```python
from build123d import *

# Parameters (mm, degrees)
SKETCH1_R           = 2.5
BOSS_EXTRUDE1_DEPTH = 1120


with BuildPart() as part:
    # Sketch1 → Boss-Extrude1 (new body)
    with BuildSketch(Plane.XY):
        with BuildLine():
            Line((2.839339828, 3.9), (-2.839339828, 3.9))
            Line((-2.839339828, 3.9), (-5.5, 6.560660172))
            Line((-5.5, 6.560660172), (-5.5, 8.2))
            Line((-5.5, 8.2), (-3.1, 8.2))
            Line((-3.1, 8.2), (-3.1, 9))
            Line((-3.1, 9), (-4.1, 10))
            Line((-4.1, 10), (-8.5, 10))
            ThreePointArc((-8.5, 10), (-9.560660172, 9.560660172), (-10, 8.5))
            Line((-10, 8.5), (-10, 4.1))
            Line((-10, 4.1), (-9, 3.1))
            Line((-9, 3.1), (-8.2, 3.1))
            Line((-8.2, 3.1), (-8.2, 5.5))
            Line((-8.2, 5.5), (-6.560660172, 5.5))
            Line((-6.560660172, 5.5), (-3.9, 2.839339828))
            Line((-3.9, 2.839339828), (-3.9, -2.839339828))
            Line((-3.9, -2.839339828), (-6.560660172, -5.5))
            Line((-6.560660172, -5.5), (-8.2, -5.5))
            Line((-8.2, -5.5), (-8.2, -3.1))
            Line((-8.2, -3.1), (-9, -3.1))
            Line((-9, -3.1), (-10, -4.1))
            Line((-10, -4.1), (-10, -8.5))
            ThreePointArc((-10, -8.5), (-9.560660172, -9.560660172), (-8.5, -10))
            Line((-8.5, -10), (-4.1, -10))
            Line((-4.1, -10), (-3.1, -9))
            Line((-3.1, -9), (-3.1, -8.2))
            Line((-3.1, -8.2), (-5.5, -8.2))
            Line((-5.5, -8.2), (-5.5, -6.560660172))
            Line((-5.5, -6.560660172), (-2.839339828, -3.9))
            Line((-2.839339828, -3.9), (2.839339828, -3.9))
            Line((2.839339828, -3.9), (5.5, -6.560660172))
            Line((5.5, -6.560660172), (5.5, -8.2))
            Line((5.5, -8.2), (3.1, -8.2))
            Line((3.1, -8.2), (3.1, -9))
            Line((3.1, -9), (4.1, -10))
            Line((4.1, -10), (8.5, -10))
            ThreePointArc((8.5, -10), (9.560660172, -9.560660172), (10, -8.5))
            Line((10, -8.5), (10, -4.1))
            Line((10, -4.1), (9, -3.1))
            Line((9, -3.1), (8.2, -3.1))
            Line((8.2, -3.1), (8.2, -5.5))
            Line((8.2, -5.5), (6.560660172, -5.5))
            Line((6.560660172, -5.5), (3.9, -2.839339828))
            Line((3.9, -2.839339828), (3.9, 2.839339828))
            Line((3.9, 2.839339828), (6.560660172, 5.5))
            Line((6.560660172, 5.5), (8.2, 5.5))
            Line((8.2, 5.5), (8.2, 3.1))
            Line((8.2, 3.1), (9, 3.1))
            Line((9, 3.1), (10, 4.1))
            Line((10, 4.1), (10, 8.5))
            ThreePointArc((10, 8.5), (9.560660172, 9.560660172), (8.5, 10))
            Line((8.5, 10), (4.1, 10))
            Line((4.1, 10), (3.1, 9))
            Line((3.1, 9), (3.1, 8.2))
            Line((3.1, 8.2), (5.5, 8.2))
            Line((5.5, 8.2), (5.5, 6.560660172))
            Line((5.5, 6.560660172), (2.839339828, 3.9))
        make_face()
        Circle(SKETCH1_R, mode=Mode.SUBTRACT)
    extrude(amount=BOSS_EXTRUDE1_DEPTH)


solid = part.part
```
Model file for the job. Use its own axes, mm. Coordinates: 2 decimals unless noted, no trailing zeros. Use a Markdown table: item, result. Add a question column.
Item 1: Two-plate mould, pull along Z, no slides. Class faces 1 (the face through (2, 2, 1120)), 2 (the face through (2, 2, 0)): pulls with the +Z half, pulls with the -Z half, needs draft (parallel to the pull), parting line crosses it, or undercut.
Item 2: Drill centre lines: line 1 along Y through (x, z) = (0, 437); line 2 along X through (y, z) = (0.5, 749.5); line 3 along X through (y, z) = (-9, 89). Where is each one in solid material? Low to high.
Item 3: Drop flat-ended pins along their axis: pin 1 (5 mm diameter, centred on y = 2.5, z = 497, fed in from +X); pin 2 (1.5 mm diameter, centred on y = -3, z = 441, fed in from +X); pin 3 (6 mm diameter, centred on y = 0.5, z = 772.5, fed in from -X); pin 4 (2 mm diameter, centred on x = -3, z = 480.5, fed in from +Y). Give the stop position or say it passes through.
A:
| question | item | result |
|---|---|---|
| 1 | face 1 | pulls with the +Z half |
| 1 | face 2 | pulls with the -Z half |
| 2 | line 1 | y = -3.9 to -2.5, 2.5 to 3.9 |
| 2 | line 2 | x = -3.9 to -2.45, 2.45 to 3.9 |
| 2 | line 3 | x = -9.91 to -3.1, 3.1 to 9.91 |
| 3 | pin 1 | stops at x = 10 |
| 3 | pin 2 | stops at x = 9.65 |
| 3 | pin 3 | stops at x = -9.4 |
| 3 | pin 4 | stops at y = 9.9 |
